from build123d import *

# Parameters (mm, degrees)
SKETCH2_W            = 30
SKETCH2_H            = 10
BOSS_EXTRUDE1_DEPTH  = 6
M3_CLEARANCE_HOLE1_D = 3.2
FILLET1_R            = 5


with BuildPart() as part:
    # Sketch2 → Boss-Extrude1 (new body)
    with BuildSketch(Plane(origin=(0, 0, 0), x_dir=(1, 0, 0), z_dir=(0, 1, 0))):
        Rectangle(SKETCH2_W, SKETCH2_H)
    extrude(amount=BOSS_EXTRUDE1_DEPTH)

    # M3 Clearance Hole1 (through all)
    with Locations(Plane(origin=(0, 6, 0), x_dir=(1, 0, 0), z_dir=(0, 1, 0))):
        with Locations((-10, 0), (10, 0)):
            Hole(M3_CLEARANCE_HOLE1_D / 2)

    # Fillet1
    fillet1_edges = [part.edges().sort_by_distance(p)[0] for p in [
        (15, 3, -5),
        (15, 3, 5),
        (-15, 3, 5),
        (-15, 3, -5),
    ]]
    fillet(fillet1_edges, radius=FILLET1_R - 0.0001)  # a hair under: the kernel refuses the full size


solid = part.part
Build history of the part. All positions in model axes, mm. Give positions to 0.01 mm unless a question says otherwise; leave off trailing zeros. Loops run counter-clockwise (first coordinate to the right, second up) from the corner with the lowest first, then second, coordinate; pieces in that order, holes last. Notation, with made-up numbers: (83.5, -11.5) - (97.5, -11.5) arc R22 ccw to (97.5, 8.5) - close; hole circle Ø2 at (70.25, 25.25). An arc over 180 degrees is marked (long way). Write item = value, one per line. Start each with the question number.
1) Band-saw the part on B-B on z = 1. Give the cut face in (x, y), plus the area to 3 significant figures.
2) Band-saw the part on D-D on z = -2. Give the cut face in (x, y), plus the area to 3 significant figures.
3) Probe probe 1 along X at (y, z) = (0.9, -1.25); probe 2 along Z at (x, y) = (-10, 2.4); probe 3 along X at (y, z) = (4.5, -0.5). List the from-to ranges inside material, lowest first. Write a range as from..to.
4) Band-saw the part on A-A on y = 2.1. Count the separate pieces of the cut face and the enclosed holes in it, plus the area to 3 significant figures.
5) Pull direction X, two halves, no side cores. Call faces 1 (the cylindrical face through (11.6, 2.96, -0.07)), 2 (the cylindrical face through (-14, 3, -3)), 3 (the flat face through (0, 3, -5)): +X half, -X half, draft (parallel to the pull), parting line (faces both ways), or undercut.
6) Drop flat-ended pins along their axis: pin 1 Ø1 at (y, z) = (4.5, -2.5) entering from -X; pin 2 Ø4 at (x, z) = (-10, 0) entering from -Y. Give the stop position or say it passes through.
7) Band-saw the part on C-C on z = -3.25. Give the cut face in (x, y).
Final values:
q1.outline = (-14.9, 0) - (-11.25, 0) - (-11.25, 6) - (-14.9, 6) - close; (-8.75, 0) - (8.75, 0) - (8.75, 6) - (-8.75, 6) - close; (11.25, 0) - (14.9, 0) - (14.9, 6) - (11.25, 6) - close
q1.area = 149 mm²
q2.outline = (-14.58, 0) - (14.58, 0) - (14.58, 6) - (-14.58, 6) - close
q2.area = 175 mm²
q3.probe_1 = -14.84..-11, -9..9, 11..14.84
q3.probe_2 = -5..-1.6, 1.6..5
q3.probe_3 = -14.97..-11.52, -8.48..8.48, 11.52..14.97
q4.separate_pieces = 1
q4.enclosed_holes = 2
q4.area = 262 mm²
q5.face_1 = undercut
q5.face_2 = -X half
q5.face_3 = draft
q6.pin_1 = -14.58
q6.pin_2 = 0
q7.outline = (-13.8, 0) - (13.8, 0) - (13.8, 6) - (-13.8, 6) - close
